Here's how the part is built. I have some questions about the finished solid (model axes, mm). A direction names the side the tool comes from. Give positions to 0.01 mm unless a question says otherwise; leave off trailing zeros. Write each loop counter-clockwise with the first axis right and the second up, starting at its lowest first coordinate (ties: lowest second). Pieces come first, ordered by that corner, then holes. Notation, with made-up numbers: (10, 89.25) -> (31, 89.25) arc R18 cw to (31, 112.25) -> close; hole circle Ø6 at (75.25, -10). An arc over 180 degrees is marked (long way). Return JSON: item names as keys, results as strings.
from build123d import *

# Parameters (mm, degrees)
SKETCH1_W               = 15
SKETCH1_H               = 8
BOSS_EXTRUDE1_DEPTH     = 10
CUT_EXTRUDE1_DEPTH      = 9
BOSS_EXTRUDE2_DEPTH     = 15
CUT_EXTRUDE2_DEPTH      = 2
SKETCH6_R               = 0.8
CUT_EXTRUDE3_DEPTH      = 9
CUT_EXTRUDE3_DEPTH_BACK = 3
FILLET1_R               = 1.5


with BuildPart() as part:
    # Sketch1 → Boss-Extrude1 (new body)
    with BuildSketch(Plane.XY):
        with Locations((0, 4)):
            Rectangle(SKETCH1_W, SKETCH1_H)
    extrude(amount=BOSS_EXTRUDE1_DEPTH)

    # Sketch2 → Cut-Extrude1 (cut, through all)
    with BuildSketch(Plane(origin=(0, 8, 0), x_dir=(1, 0, 0), z_dir=(0, 1, 0))):
        with BuildLine():
            Line((-1.25, -2), (1.25, -2))
            ThreePointArc((1.25, -2), (2.204594155, -2.395405845), (2.6, -3.35))
            Line((2.6, -3.35), (2.6, -8.35))
            ThreePointArc((2.6, -8.35), (2.204594155, -9.304594155), (1.25, -9.7))
            Line((1.25, -9.7), (-1.25, -9.7))
            ThreePointArc((-1.25, -9.7), (-2.204594155, -9.304594155), (-2.6, -8.35))
            Line((-2.6, -8.35), (-2.6, -3.35))
            ThreePointArc((-2.6, -3.35), (-2.204594155, -2.395405845), (-1.25, -2))
        make_face()
    extrude(amount=-CUT_EXTRUDE1_DEPTH, mode=Mode.SUBTRACT)

    # Sketch3 → Boss-Extrude2 (add)
    with BuildSketch(Plane(origin=(-7.5, 0, 0), x_dir=(0, 0, -1), z_dir=(1, 0, 0))):
        with BuildLine():
            ThreePointArc((-18.235493239, 8), (-16.655013859, 2.966168092), (-14.873286259, -2))
            Line((-14.873286259, -2), (0, -2))
            Line((0, -2), (0, 0))
            Line((0, 0), (-10, 0))
            Line((-10, 0), (-10, 8))
            Line((-10, 8), (-15.107085438, 8))
            Line((-15.107085438, 8), (-18.235493239, 8))
        make_face()
    extrude(amount=BOSS_EXTRUDE2_DEPTH)

    # Sketch5 → Cut-Extrude2 (cut)
    with BuildSketch(Plane(origin=(7.5, 0, 0), x_dir=(0, 0, -1), z_dir=(1, 0, 0))):
        with BuildLine():
            Line((0, 1), (-11, 1))
            ThreePointArc((-11, 1), (-12.25, 2.25), (-11, 3.5))
            Line((-11, 3.5), (0, 3.5))
            Line((0, 3.5), (0, 1))
        make_face()
    cut_extrude2 = extrude(amount=-CUT_EXTRUDE2_DEPTH, mode=Mode.SUBTRACT)

    # Mirror1: Cut-Extrude2 across plane
    add(cut_extrude2.mirror(Plane(origin=(0, 0, 0), x_dir=(0, 0, 1), z_dir=(1, 0, 0))), mode=Mode.SUBTRACT)

    # Sketch6 → Cut-Extrude3 (cut, two sides)
    with BuildSketch(Plane(origin=(0, 0, 0), x_dir=(1, 0, 0), z_dir=(0, 1, 0))) as cut_extrude3_sk:
        with Locations((-1.25, -3.35)):
            Circle(SKETCH6_R)
        with Locations((1.25, -3.35)):
            Circle(SKETCH6_R)
        with Locations((1.25, -5.85)):
            Circle(SKETCH6_R)
        with Locations((1.25, -8.35)):
            Circle(SKETCH6_R)
        with Locations((-1.25, -5.85)):
            Circle(SKETCH6_R)
        with Locations((-1.25, -8.35)):
            Circle(SKETCH6_R)
    extrude(amount=CUT_EXTRUDE3_DEPTH, mode=Mode.SUBTRACT)
    extrude(cut_extrude3_sk.sketch, amount=-CUT_EXTRUDE3_DEPTH_BACK, mode=Mode.SUBTRACT)

    # Fillet1
    fillet1_edges = [part.edges().sort_by_distance(p)[0] for p in [
        (-7.5, -2, 7.436643129),
        (0, -2, 14.873286259),
        (-7.5, 2.966168092, 16.655013859),
        (0, 8, 18.235493239),
        (7.5, 2.966168092, 16.655013859),
        (7.5, -2, 7.436643129),
        (-7.5, 8, 9.11774662),
        (7.5, 8, 9.11774662),
    ]]
    fillet(fillet1_edges, radius=FILLET1_R)


solid = part.part
1. Suppose I cut it at A-A, the plane z = 5.85. List the corners of the cut face in (x, y) for me, and give its area (3 significant figures).
Taken from the geometry:
{"outline": "(-7.5, -0.5) arc R1.5 ccw to (-6, -2) -> (-2.05, -2) -> (-2.05, 0) -> (-2.6, 0) -> (-2.6, 8) -> (-6, 8) arc R1.5 ccw to (-7.5, 6.5) -> (-7.5, 3.5) -> (-5.5, 3.5) -> (-5.5, 1) -> (-7.5, 1) -> close; (-0.45, -2) -> (0.45, -2) -> (0.45, 0) -> (-0.45, 0) -> close; (2.05, -2) -> (6, -2) arc R1.5 ccw to (7.5, -0.5) -> (7.5, 1) -> (5.5, 1) -> (5.5, 3.5) -> (7.5, 3.5) -> (7.5, 6.5) arc R1.5 ccw to (6, 8) -> (2.6, 8) -> (2.6, 0) -> (2.05, 0) -> close", "area": "90.1 mm²"}
2. Suppose I cut it at C-C, the plane z = 10.75. List the corners of the cut face in (x, y) for me.
Taken from the geometry:
{"outline": "(-7.5, -0.5) arc R1.5 ccw to (-6, -2) -> (6, -2) arc R1.5 ccw to (7.5, -0.5) -> (7.5, 1) -> (5.5, 1) -> (5.5, 3.5) -> (7.5, 3.5) -> (7.5, 6.5) arc R1.5 ccw to (6, 8) -> (-6, 8) arc R1.5 ccw to (-7.5, 6.5) -> (-7.5, 3.5) -> (-5.5, 3.5) -> (-5.5, 1) -> (-7.5, 1) -> close"}
3. If I drill on line 1 (X direction, y = -0.4, z = 3.35); line 2 (X direction, y = -1.2, z = 3.35); line 3 (Z direction, x = -1.25, y = -0.6), over which ranges is the centre line in solid material (lowest first)? Write a range as [from, to].
Taken from the geometry:
{"line 1": "x = [-7.5, -2.05], [-0.45, 0.45], [2.05, 7.5]", "line 2": "x = [-7.33, -2.05], [-0.45, 0.45], [2.05, 7.33]", "line 3": "z = [0, 2.55], [4.15, 5.05], [6.65, 7.55], [9.15, 15.4]"}
4. Suppose I cut it at D-D, the plane z = 8.75. List the corners of the cut face in (x, y) for me.
Taken from the geometry:
{"outline": "(-7.5, -0.5) arc R1.5 ccw to (-6, -2) -> (-1.94, -2) -> (-1.94, 0) -> (-2.54, 0) -> (-2.54, 8) -> (-6, 8) arc R1.5 ccw to (-7.5, 6.5) -> (-7.5, 3.5) -> (-5.5, 3.5) -> (-5.5, 1) -> (-7.5, 1) -> close; (-0.56, -2) -> (0.56, -2) -> (0.56, 0) -> (-0.56, 0) -> close; (1.94, -2) -> (6, -2) arc R1.5 ccw to (7.5, -0.5) -> (7.5, 1) -> (5.5, 1) -> (5.5, 3.5) -> (7.5, 3.5) -> (7.5, 6.5) arc R1.5 ccw to (6, 8) -> (2.54, 8) -> (2.54, 0) -> (1.94, 0) -> close"}
5. For pin 1 Ø2.5 at (x, z) = (0, 6.5) entering from +Y; pin 2 Ø0.8 at (y, z) = (2, 3.5) entering from +X; pin 3 Ø1.2 at (x, y) = (0, 5.5) entering from +Z; pin 4 Ø1 at (x, z) = (1.25, 5.85) entering from +Y, each with a flat end and sliding along its axis, tell me the tip position at first contact or that it passes through.
Taken from the geometry:
{"pin 1": "stops at y = 0", "pin 2": "stops at x = 5.5", "pin 3": "stops at z = 17.66", "pin 4": "passes through"}
6. If we mould it in two halves opening along X, with no side actions, what happens to faces 1 (the face through (0, 4, 2)), 2 (the face through (7.05, -1.57, 6.82)), 3 (the face through (-0.084, 2.549, 16.514))? For each: released by +X, released by -X, zero draft, split by the parting line, or undercut.
Taken from the geometry:
{"face 1": "undercut", "face 2": "released by +X", "face 3": "zero draft"}
7. Which directions (+Z, -Z, +X, -X, +Y, -Y) give clear straight access to the entire face, cutting with the end or side of a thin tool? Please do faces 4 (the face through (-7.05, 7.57, 8.22)), 5 (the face through (2.19, 4.06, 2.38)), 6 (the face through (6.51, 2.22, 12.25)).
Taken from the geometry:
{"face 4": "+Z, -Z, -X, +Y", "face 5": "+Y", "face 6": "-Z, +X"}
8. Suppose I cut it at B-B, the plane x = 5.75. List the corners of the cut face in (y, z) for me, and give its area (3 significant figures).
Taken from the geometry:
{"outline": "(-2, 0) -> (1, 0) -> (1, 11) arc R1.25 cw to (3.5, 11) -> (3.5, 0) -> (8, 0) -> (8, 16.22) arc R1.5 ccw to (6.06, 17.65) arc R131.11 ccw to (-1.02, 15.24) arc R1.5 ccw to (-2, 13.84) -> close", "area": "135 mm²"}
